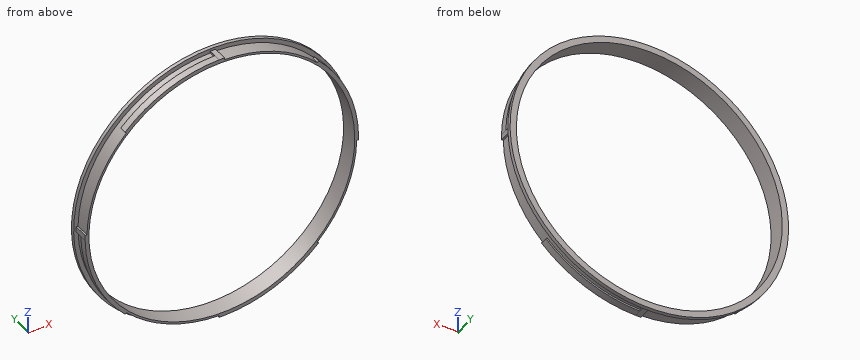
from build123d import *

# Parameters (mm, degrees)
SKETCH_1_R      = 74.6
SKETCH_1_R_2    = 73.5
EXTRUDE_1_DEPTH = 10
SKETCH_2_W      = 1
SKETCH_2_H      = 3
SKETCH_2_W_2    = 3
SKETCH_2_H_2    = 1
EXTRUDE_2_DEPTH = 10
EXTRUDE_4_DEPTH = 3.9
EXTRUDE_START   = -2
SKETCH_4_R      = 77
SKETCH_4_R_2    = 74.6
EXTRUDE_5_DEPTH = 2


with BuildPart() as part:
    # 草图1 → 凸台-拉伸1 (new body)
    with BuildSketch(Plane(origin=(0, 0, 0), x_dir=(1, 0, 0), z_dir=(0, 1, 0))):
        with Locations(Location((0, 0, 0), (0, 0, 270))):
            Circle(SKETCH_1_R)
        with Locations(Location((0, 0, 0), (0, 0, 270))):
            Circle(SKETCH_1_R_2, mode=Mode.SUBTRACT)
    extrude(amount=EXTRUDE_1_DEPTH)

    # 草图2 → 凸台-拉伸2 (add)
    with BuildSketch(Plane(origin=(0, 0, 0), x_dir=(1, 0, 0), z_dir=(0, 1, 0))):
        with Locations((75.084918046, 0)):
            Rectangle(SKETCH_2_W, SKETCH_2_H)
        with Locations((0, -75.084918046)):
            Rectangle(SKETCH_2_W_2, SKETCH_2_H_2)
        with Locations((-75.084918046, 0)):
            Rectangle(SKETCH_2_W, SKETCH_2_H)
        with Locations((0, 75.084918046)):
            Rectangle(SKETCH_2_W_2, SKETCH_2_H_2)
    extrude(amount=EXTRUDE_2_DEPTH)

    # 草图3 → 凸台-拉伸4 (add)
    with BuildSketch(Plane(origin=(0, 0, 0), x_dir=(1, 0, 0), z_dir=(0, 1, 0))):
        with BuildLine():
            ThreePointArc((53.457131592, 53.457131592), (29.622311043, 69.554644162), (1.5, 75.584918046))
            Line((1.5, 75.584918046), (1.5, 74.584918046))
            ThreePointArc((1.5, 74.584918046), (29.239685788, 68.630902478), (52.750165877, 52.750165877))
            Line((52.750165877, 52.750165877), (53.457131592, 53.457131592))
        make_face()
        with BuildLine():
            Line((52.750165877, -52.750165877), (53.457131592, -53.457131592))
            ThreePointArc((53.457131592, -53.457131592), (69.554644162, -29.622311043), (75.584918046, -1.5))
            Line((75.584918046, -1.5), (74.584918046, -1.5))
            ThreePointArc((74.584918046, -1.5), (68.630902478, -29.239685788), (52.750165877, -52.750165877))
        make_face()
        with BuildLine():
            Line((-52.750165877, -52.750165877), (-53.457131592, -53.457131592))
            ThreePointArc((-53.457131592, -53.457131592), (-29.622311043, -69.554644162), (-1.5, -75.584918046))
            Line((-1.5, -75.584918046), (-1.5, -74.584918046))
            ThreePointArc((-1.5, -74.584918046), (-29.239685788, -68.630902478), (-52.750165877, -52.750165877))
        make_face()
        with BuildLine():
            Line((-52.750165877, 52.750165877), (-53.457131592, 53.457131592))
            ThreePointArc((-53.457131592, 53.457131592), (-69.554644162, 29.622311043), (-75.584918046, 1.5))
            Line((-75.584918046, 1.5), (-74.584918046, 1.5))
            ThreePointArc((-74.584918046, 1.5), (-68.630902478, 29.239685788), (-52.750165877, 52.750165877))
        make_face()
    extrude(amount=EXTRUDE_4_DEPTH)

    # 草图4 → 凸台-拉伸5 (add)
    with BuildSketch(Plane(origin=(0, 10, 0), x_dir=(1, 0, 0), z_dir=(0, 1, 0)).offset(EXTRUDE_START)):
        with Locations(Location((0, 0, 0), (0, 0, 270))):
            Circle(SKETCH_4_R)
        Circle(SKETCH_4_R_2, mode=Mode.SUBTRACT)
    extrude(amount=EXTRUDE_5_DEPTH)


solid = part.part
Read the model definition and answer for the solid it produces. Units are mm, in the model's axes. Round coordinates to 2 decimals unless told otherwise and drop trailing zeros. Order: outer loops, then holes, each group sorted by start corner. A loop starts at its lowest first (then second) coordinate and runs counter-clockwise, first axis right, second up. Notation, with made-up numbers: (5.25, -37.75) - (13.25, -37.75) arc R11 ccw to (13.25, -29.75) - close; hole circle Ø5 at (59.25, 74). An arc over 180 degrees is marked (long way). Use one line per item in the form item = value. Start each with the question number.
(1) The part is cut by section B-B (x = 50.5). Give the vertices of the cut face in (y, z), then the cut area to 3 significant figures.
(2) The part is cut by section A-A (y = 6.25). Give the vertices of the cut face in (x, z), then the cut area to 3 significant figures.
(3) Flat-ended cylindrical pins translate along their axes: pin 1 Ø2 at (y, z) = (1.5, 22.5) entering from +X; pin 2 Ø0.8 at (y, z) = (4.5, -75.5) entering from -X; pin 3 Ø1.5 at (x, y) = (-52.5, 7.5) entering from -Z; pin 4 Ø18.5 at (x, z) = (-17.5, 61.5) entering from +Y. Find the tip coordinate at first contact, or state that the pin passes through.
(4) Find the intervals of material crossed by line 1 along X through (y, z) = (4.5, 0); line 2 along Z through (x, y) = (60.5, 8.5); line 3 along X through (y, z) = (6.25, -30.5), in increasing order. Write a range as from..to.
(5) The part is cut by section C-C (z = 33.5). Give the vertices of the cut face in (x, y).
Checked values:
q1.outline = (0, -56.26) - (3.9, -56.26) - (3.9, -54.91) - (8, -54.91) - (8, -58.13) - (10, -58.13) - (10, -53.4) - (0, -53.4) - close; (0, 53.4) - (10, 53.4) - (10, 58.13) - (8, 58.13) - (8, 54.91) - (0, 54.91) - close
q1.area = 48.2 mm^2
q2.outline = (-75.58, -1.5) - (-74.58, -1.5) arc R74.6 ccw to (-1.5, -74.58) - (-1.5, -75.58) - (1.5, -75.58) - (1.5, -74.58) arc R74.6 ccw to (74.58, -1.5) - (75.58, -1.5) - (75.58, 1.5) - (74.58, 1.5) arc R74.6 ccw to (1.5, 74.58) - (1.5, 75.58) - (-1.5, 75.58) - (-1.5, 74.58) arc R74.6 ccw to (-74.58, 1.5) - (-75.58, 1.5) - close; hole circle Ø147 at (0, 0)
q2.area = 524 mm^2
q3.pin_1 = 72.48
q3.pin_2 = -1.5
q3.pin_3 = -56.84
q3.pin_4 = through
q4.line_1 = -75.58..-73.5, 73.5..75.58
q4.line_2 = -47.63..-41.74, 41.74..47.63
q4.line_3 = -68.08..-66.87, 66.87..68.08
q5.outline = (-69.33, 8) - (-66.66, 8) - (-66.66, 0) - (-65.42, 0) - (-65.42, 10) - (-69.33, 10) - close; (65.42, 0) - (67.77, 0) - (67.77, 3.9) - (66.66, 3.9) - (66.66, 8) - (69.33, 8) - (69.33, 10) - (65.42, 10) - close
